from build123d import *

# Parameters (mm, degrees)
F0_R     = 14.2875
F1_DEPTH = 6.35
F2_DEPTH = 101.6


with BuildPart() as f1:
    # F0 (on Front) → F1 (new body)
    with BuildSketch(Plane.XZ):
        with BuildLine():
            Line((327.579371, -271.476441), (362.607836, -298.86714))
            ThreePointArc((362.607836, -298.86714), (0, 469.9), (-362.607836, -298.86714))
            Line((-362.607836, -298.86714), (-327.579371, -271.476441))
            ThreePointArc((-327.579371, -271.476441), (0, 425.45), (327.579371, -271.476441))
        make_face()
        with Locations((-432.420844, -115.866816)):
            Circle(F0_R, mode=Mode.SUBTRACT)
        with Locations((432.420844, -115.866816)):
            Circle(F0_R, mode=Mode.SUBTRACT)
        with Locations((-432.420844, 115.866816)):
            Circle(F0_R, mode=Mode.SUBTRACT)
        with Locations((-316.554028, 316.554028)):
            Circle(F0_R, mode=Mode.SUBTRACT)
        with Locations((-115.866816, 432.420844)):
            Circle(F0_R, mode=Mode.SUBTRACT)
        with Locations((432.420844, 115.866816)):
            Circle(F0_R, mode=Mode.SUBTRACT)
        with Locations((115.866816, 432.420844)):
            Circle(F0_R, mode=Mode.SUBTRACT)
        with Locations((316.554028, 316.554028)):
            Circle(F0_R, mode=Mode.SUBTRACT)
    extrude(amount=F1_DEPTH)

    # F0 (on Front) → F2 (join)
    with BuildSketch(Plane.XZ):
        with BuildLine():
            Line((322.575083, -267.563312), (327.579371, -271.476441))
            ThreePointArc((327.579371, -271.476441), (0, 425.45), (-327.579371, -271.476441))
            Line((-327.579371, -271.476441), (-322.575083, -267.563312))
            ThreePointArc((-322.575083, -267.563312), (0, 419.1), (322.575083, -267.563312))
        make_face()
    extrude(amount=F2_DEPTH)


solid = f1.part
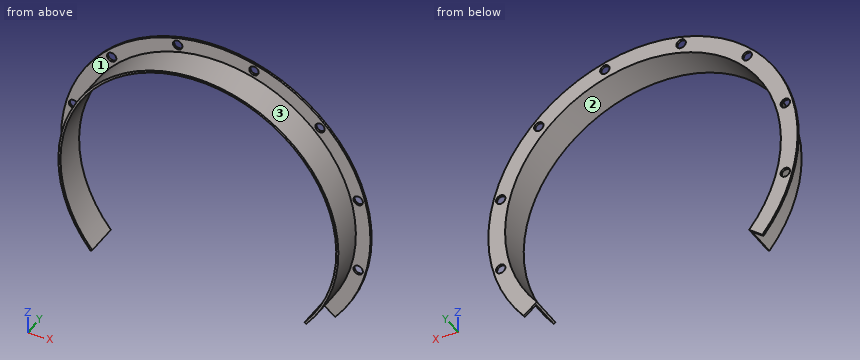
The listing builds one solid part. Answer for the finished solid, in the listing's coordinates (mm). Face numbers are marked on the shaded views. Give positions to 0.01 mm unless a question says otherwise; leave off trailing zeros. Loops run counter-clockwise (first coordinate to the right, second up) from the corner with the lowest first, then second, coordinate; pieces in that order, holes last.
Item 1: A cutting plane is placed at D-D (x = 0). Give the vertices of the cut face in (y, z), then the cut area to 3 significant figures.
Derived:
outline: (-101.6, 419.1) - (0, 419.1) - (0, 469.9) - (-6.35, 469.9) - (-6.35, 425.45) - (-101.6, 425.45) - close
area: 927 mm2
Item 2: A cutting plane is placed at C-C (y = -63). Give the vertices of the cut face in (x, z), then the cut area to 3 significant figures.
Derived:
outline: (-327.58, -271.48) - (-322.58, -267.56) arc R419.1 cw (long way) to (322.58, -267.56) - (327.58, -271.48) arc R425.45 ccw (long way) to start
area: 12,100 mm2
Item 3: A cutting plane is placed at A-A (z = 0). Give the vertices of the cut face in (x, y).
Derived:
outline: (-469.9, -6.35) - (-425.45, -6.35) - (-425.45, -101.6) - (-419.1, -101.6) - (-419.1, 0) - (-469.9, 0) - close; (419.1, -101.6) - (425.45, -101.6) - (425.45, -6.35) - (469.9, -6.35) - (469.9, 0) - (419.1, 0) - close
Item 4: Find the intervals of material crossed by line 1 along X through (y, z) = (-40, 8); line 2 along X through (y, z) = (-47.5, 0); line 3 along Y through (x, z) = (-138, 407), in increasing order.
Derived:
line 1: x = -425.37 to -419.02, 419.02 to 425.37
line 2: x = -425.45 to -419.1, 419.1 to 425.45
line 3: y = -6.35 to 0
Item 5: Determine the mould class of the marked faces 1, 2 and 3 for opening direction Z: +Z half, -Z half, draft (parallel to the pull), parting line (faces both ways), or undercut.
Derived:
face 1: draft
face 2: undercut
face 3: parting line
Item 6: A cutting plane is placed at B-B (x = -115). Give the vertices of the cut face in (y, z), then the cut area to 3 significant figures.
Derived:
outline: (-101.6, 403.01) - (0, 403.01) - (0, 418.16) - (-6.35, 418.16) - (-6.35, 409.61) - (-101.6, 409.61) - close; (-6.35, 446.68) - (0, 446.68) - (0, 455.61) - (-6.35, 455.61) - close
area: 781 mm2
Item 7: Each of these flat-tipped pins is pushed along its axis until it touches: pin 1 Ø12 at (y, z) = (-60, 205) entering from +X; pin 2 Ø8 at (x, y) = (277.5, -62.5) entering from +Z; pin 3 Ø3 at (y, z) = (-80, 195.5) entering from +X. Where does it stop, or does it pass through?
Derived:
pin 1: stops at x = 376.04
pin 2: stops at z = 325.89
pin 3: stops at x = 378.64
